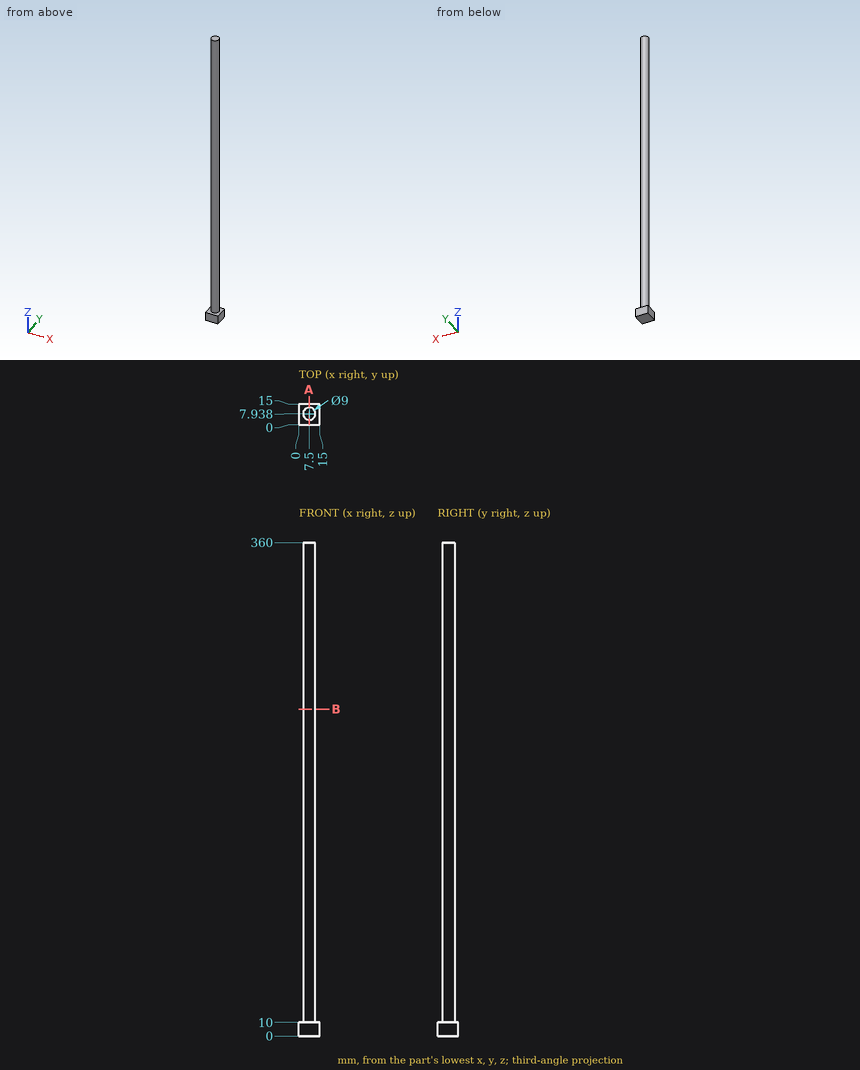
Verification items for this drawing (mm, ordinates from the low corner). Coordinates: 2 decimals unless noted, no trailing zeros. Order: outer loops, then holes, each group sorted by start corner. A loop starts at its lowest first (then second) coordinate and runs counter-clockwise, first axis right, second up. Notation, with made-up numbers: (64.25, 0) - (96.25, 0) arc R13 cw to (96.25, 6) - close; hole circle Ø7 at (2.25, 55). An arc over 180 degrees is marked (long way). Answer in a Markdown table with one row per item. Add a question column.
1. Gauge pin test, flat ends, axial feed: pin 1 Ø1 at (x, z) = (8.5, 219.5) entering from +Y; pin 2 Ø1 at (y, z) = (12, 240.5) entering from +X; pin 3 Ø6 at (y, z) = (9.5, 308) entering from +X. Record the tip position at first contact, or that the pin passes through.
2. Section check A-A (x = 7.5). Enter the section's corners in (y, z), plus the area to 3 significant figures.
3. Material ranges on L1, parallel to Y at x = 7, z = 233.5 (1 decimal); L2, parallel to Z at x = 6, y = 14; L3, parallel to Y at x = 7.5, z = 342.5, recorded low to high. Write a range as [from, to].
4. Section check B-B (z = 238.5). Enter the section's corners in (x, y), plus the area to 3 significant figures.
Data:
| question | item | result |
|---|---|---|
| 1 | pin 1 | stops at y = 12.41 |
| 1 | pin 2 | stops at x = 10.25 |
| 1 | pin 3 | stops at x = 12 |
| 2 | outline | (0, 0) - (15, 0) - (15, 10) - (12.44, 10) - (12.44, 360) - (3.44, 360) - (3.44, 10) - (0, 10) - close |
| 2 | area | 3,300 mm² |
| 3 | L1 | y = [3.5, 12.4] |
| 3 | L2 | z = [0, 10] |
| 3 | L3 | y = [3.44, 12.44] |
| 4 | outline | circle Ø9 at (7.5, 7.94) |
| 4 | area | 63.6 mm² |
